Geometry check sheet. Reference: drawing and pictorial views, mm from the part's lowest x, y, z. A direction names the side the tool comes from. Give positions to 0.01 mm unless a question says otherwise; leave off trailing zeros. Order: outer loops, then holes, each group sorted by start corner. A loop starts at its lowest first (then second) coordinate and runs counter-clockwise, first axis right, second up. Notation, with made-up numbers: M 57.25,52 L 83.25,52 A29 ccw 83.25,89 Z; hole C 4.5,-23.75 d5. An arc over 180 degrees is marked long. Answer as a JSON object with one key per item and string values. Group by question number.
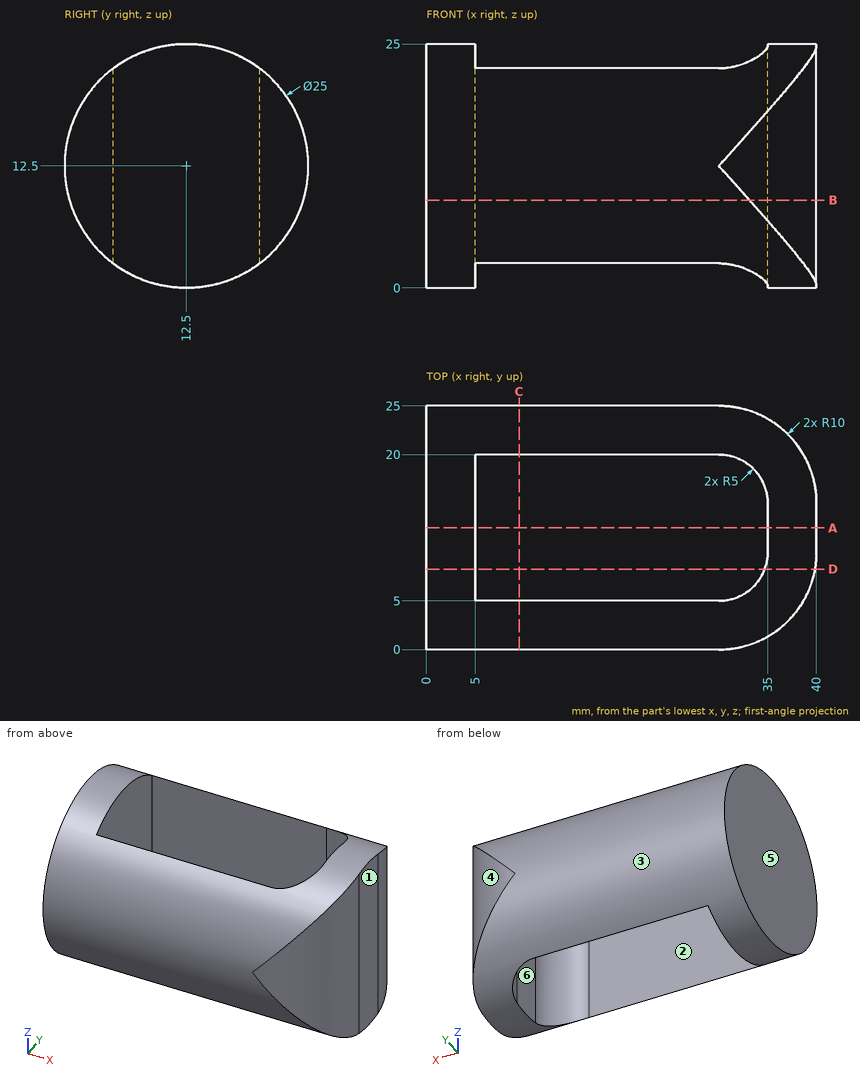
1. Cross-section at C-C (x = 9.5). Record the cut outline in (y, z).
2. Cross-section at D-D (y = 8.25). Record the cut outline in (x, z).
3. Thickness scan on line 1 along Y through (x, z) = (28, 12); line 2 along X through (y, z) = (11.5, 10.25); line 3 along X through (y, z) = (8.5, 16.5). Record the ranges inside material, lowest first. Write a range as [from, to].
4. Cross-section at B-B (z = 9). Record the cut outline in (x, y), and give its area (3 significant figures).
5. Release check for a two-part mould opening along Y. For the marked faces 1, 2, 3 and 4 record: released by +Y, released by -Y, zero draft, split by the parting line, or undercut.
6. Access from +Z, -Z, +X, -X, +Y, -Y to the whole of each face (thin tool, end or side, straight path). Record for the marked faces 5 and 6.
7. Depth check by flat-ended pin: pin 1 (2 mm diameter, centred on x = 13, y = 7, fed in from +Z); pin 2 (4 mm diameter, centred on x = 20.5, z = 3, fed in from +Y); pin 3 (1.5 mm diameter, centred on y = 19.5, z = 13.5, fed in from +X); pin 4 (5 mm diameter, centred on x = 31, z = 7.5, fed in from -Y). Enter the tip coordinate at first touch or a pass-through.
8. Cross-section at A-A (y = 12.5). Record the cut outline in (x, z).
Report:
{
 "1": {"outline": "M 5,2.5 L 5,22.5 A12.5 ccw Z; M 20,2.5 A12.5 ccw 20,22.5 Z"},
 "2": {"outline": "M 0,0.74 L 5,0.74 L 5,24.26 L 0,24.26 Z; M 34.68,0.74 L 39.85,0.74 L 39.85,24.26 L 34.68,24.26 Z"},
 "3": {"line 1": "y = [0.01, 5], [20, 24.99]", "line 2": "x = [0, 5], [35, 40]", "line 3": "x = [0, 5], [34.77, 39.89]"},
 "4": {"outline": "M 0,0.5 L 33.12,0.5 A10 ccw 40,10 L 40,15 A10 ccw 33.12,24.5 L 0,24.5 Z; hole M 5,5 L 30,5 A5 ccw 35,10 L 35,15 A5 ccw 30,20 L 5,20 Z", "area": "486 mm2"},
 "5": {"face 1": "zero draft", "face 2": "undercut", "face 3": "split by the parting line", "face 4": "released by +Y"},
 "6": {"face 5": "+Z, -Z, -X, +Y, -Y", "face 6": "+Z, -Z"},
 "7": {"pin 1": "passes through", "pin 2": "stops at y = 22.5", "pin 3": "stops at x = 39.27", "pin 4": "stops at y = 0.25"},
 "8": {"outline": "M 0,0 L 5,0 L 5,25 L 0,25 Z; M 35,0 L 40,0 L 40,25 L 35,25 Z"}
}
